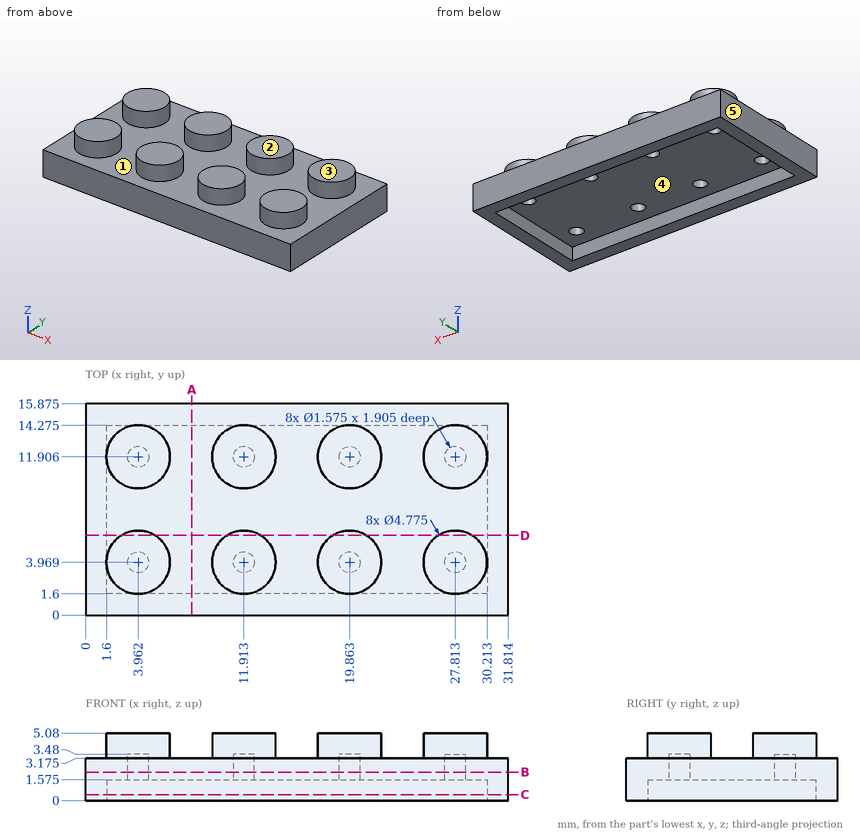
Could you check a few things on this drawing? It's one solid part, dimensions in mm from its lowest x, y, z. A direction names the side the tool comes from. Round coordinates to 2 decimals unless told otherwise and drop trailing zeros. Write each loop counter-clockwise with the first axis right and the second up, starting at its lowest first coordinate (ties: lowest second). Pieces come first, ordered by that corner, then holes. Notation, with made-up numbers: (32.25, 84) -> (82.25, 84) arc R24 cw to (82.25, 112) -> close; hole circle Ø8 at (-4, 35.5). An arc over 180 degrees is marked (long way). One line per item, written item: value.
1) For the marked faces 1 and 2, which set-ups out of +Z, -Z, +X, -X, +Y, -Y let a thin tool reach every point of the face, with its end or its side?
Filled sheet:
face 1: +Z
face 2: +Z, +X, -X, +Y, -Y
2) I'm going to push flat-ended pins straight in: pin 1 Ø0.9 at (x, y) = (27.81, 3.97) entering from -Z; pin 2 Ø1.7 at (x, y) = (19.5, 11.5) entering from -Z (1 decimal); pin 3 Ø3 at (x, y) = (27, 8) entering from +Z (1 decimal). Where does each tip first touch, or does it pass through?
Filled sheet:
pin 1: stops at z = 3.48
pin 2: stops at z = 1.6
pin 3: stops at z = 3.2
3) Suppose I cut it at C-C on z = 0.45. List the corners of the cut face in (x, y) for me (1 decimal).
Filled sheet:
outline: (0, 0) -> (31.8, 0) -> (31.8, 15.9) -> (0, 15.9) -> close; hole (1.6, 1.6) -> (30.2, 1.6) -> (30.2, 14.3) -> (1.6, 14.3) -> close
4) Suppose I cut it at B-B on z = 2.15. Give the number of separate pieces and of enclosed holes in the cut face.
Filled sheet:
separate pieces: 1
enclosed holes: 8
5) If I drill on line 1 (X direction, y = 2.75, z = 0.3); line 2 (X direction, y = 3.5, z = 4) (1 decimal); line 3 (Y direction, x = 29.5, z = 0.75) (1 decimal), over which ranges is the centre line in solid material (lowest first)? Write a range as [from, to].
Filled sheet:
line 1: x = [0, 1.6], [30.21, 31.81]
line 2: x = [1.6, 6.3], [9.6, 14.3], [17.5, 22.2], [25.5, 30.2]
line 3: y = [0, 1.6], [14.3, 15.9]
6) We'd pull the mould along X, two halves only. Please class the marked faces 3, 4 and 5: released by +X, released by -X, zero draft, split by the parting line, or undercut.
Filled sheet:
face 3: zero draft
face 4: undercut
face 5: released by -X
7) Suppose I cut it at D-D on y = 6. List the corners of the cut face in (x, z) for me (1 decimal).
Filled sheet:
outline: (0, 0) -> (1.6, 0) -> (1.6, 1.6) -> (30.2, 1.6) -> (30.2, 0) -> (31.8, 0) -> (31.8, 3.2) -> (29.1, 3.2) -> (29.1, 5.1) -> (26.6, 5.1) -> (26.6, 3.2) -> (21.1, 3.2) -> (21.1, 5.1) -> (18.6, 5.1) -> (18.6, 3.2) -> (13.2, 3.2) -> (13.2, 5.1) -> (10.7, 5.1) -> (10.7, 3.2) -> (5.2, 3.2) -> (5.2, 5.1) -> (2.7, 5.1) -> (2.7, 3.2) -> (0, 3.2) -> close
8) Suppose I cut it at A-A on x = 8. List the corners of the cut face in (y, z) for me (1 decimal).
Filled sheet:
outline: (0, 0) -> (1.6, 0) -> (1.6, 1.6) -> (14.3, 1.6) -> (14.3, 0) -> (15.9, 0) -> (15.9, 3.2) -> (0, 3.2) -> close
